Design review of the part built by this model. Coordinates are the model's own, in mm. Face numbers are marked on the shaded views. A direction names the side the tool comes from. Give positions to 0.01 mm unless a question says otherwise; leave off trailing zeros. Write each loop counter-clockwise with the first axis right and the second up, starting at its lowest first coordinate (ties: lowest second). Pieces come first, ordered by that corner, then holes. Notation, with made-up numbers: M -2.75,-17 L 27.25,-17 A23 ccw 27.25,21 Z; hole C 35,-21.5 d11. An arc over 180 degrees is marked long. Write each question's results on one line, items separated by ' | '. Start each with the question number.
from build123d import *

# Parameters (mm, degrees)
SKETCH1_W           = 20
SKETCH1_H           = 20
BOSS_EXTRUDE1_DEPTH = 6
SKETCH2_W           = 6.8
SKETCH2_H           = 20
BOSS_EXTRUDE2_DEPTH = 6
SKETCH3_W           = 7
SKETCH3_H           = 20
BOSS_EXTRUDE3_DEPTH = 15
CHAMFER1_SIZE       = 6
SKETCH4_R           = 3
CUT_EXTRUDE1_DEPTH  = 10
SKETCH5_W           = 20
SKETCH5_H           = 20
BOSS_EXTRUDE4_DEPTH = 18
CUT_EXTRUDE2_DEPTH  = 2
SKETCH9_W           = 20
SKETCH9_H           = 8.1
BOSS_EXTRUDE5_DEPTH = 23
CUT_EXTRUDE5_REACH  = 54.058
SKETCH10_R          = 3
SKETCH11_R          = 5.05
CUT_EXTRUDE6_DEPTH  = 6.1


with BuildPart() as part:
    # Sketch1 → Boss-Extrude1 (new body)
    with BuildSketch(Plane(origin=(0, 0, 0), x_dir=(1, 0, 0), z_dir=(0, 1, 0))):
        Rectangle(SKETCH1_W, SKETCH1_H)
    extrude(amount=BOSS_EXTRUDE1_DEPTH)

    # Sketch2 → Boss-Extrude2 (add)
    with BuildSketch(Plane(origin=(0, 6, 0), x_dir=(1, 0, 0), z_dir=(0, 1, 0))):
        with Locations((6.6, 0)):
            Rectangle(SKETCH2_W, SKETCH2_H)
    extrude(amount=BOSS_EXTRUDE2_DEPTH)

    # Sketch3 → Boss-Extrude3 (add)
    with BuildSketch(Plane(origin=(0, 6, 0), x_dir=(1, 0, 0), z_dir=(0, 1, 0))):
        with Locations((-6.5, 0)):
            Rectangle(SKETCH3_W, SKETCH3_H)
    extrude(amount=BOSS_EXTRUDE3_DEPTH)

    # Chamfer1
    chamfer1_edges = [part.edges().sort_by_distance(p)[0] for p in [
        (-10, 21, 0),
    ]]
    chamfer(chamfer1_edges, length=CHAMFER1_SIZE)

    # Sketch4 → Cut-Extrude1 (cut)
    with BuildSketch(Plane(origin=(-12.5, 12.5, 0), x_dir=(0, 0, 1), z_dir=(-0.7071067811865489, 0.7071067811865462, 0))):
        with Locations(Location((0, 7.432512212, 0), (0, 0, 270))):
            Circle(SKETCH4_R)
    extrude(amount=-CUT_EXTRUDE1_DEPTH, mode=Mode.SUBTRACT)

    # Sketch5 → Boss-Extrude4 (add)
    with BuildSketch(Plane.XZ):
        Rectangle(SKETCH5_W, SKETCH5_H)
    extrude(amount=BOSS_EXTRUDE4_DEPTH)

    # Sketch6 → Cut-Extrude2 (cut)
    with BuildSketch(Plane(origin=(-12.5, 12.5, 0), x_dir=(0, 0, 1), z_dir=(-0.7071067811865489, 0.7071067811865462, 0))):
        Polygon((0, 13.8411002), (-5.55, 10.636806206), (-5.55, 4.228218218), (0, 1.023924224), (5.55, 4.228218218), (5.55, 10.636806206), align=None)
    extrude(amount=-CUT_EXTRUDE2_DEPTH, mode=Mode.SUBTRACT)

    # Sketch9 → Boss-Extrude5 (add)
    with BuildSketch(Plane(origin=(10, 0, 0), x_dir=(0, 0, -1), z_dir=(1, 0, 0))):
        with Locations((0, -13.95)):
            Rectangle(SKETCH9_W, SKETCH9_H)
    boss_extrude5 = extrude(amount=BOSS_EXTRUDE5_DEPTH)

    # Sketch10 → Cut-Extrude5 (cut, up to next)
    with BuildSketch(Plane.XZ.offset(18), mode=Mode.PRIVATE) as cut_extrude5_sk1:
        with Locations(Location((25, 0, 0), (0, 0, 270))):
            Circle(SKETCH10_R)
    cut_extrude5_tool1 = extrude(cut_extrude5_sk1.sketch, amount=-CUT_EXTRUDE5_REACH, mode=Mode.PRIVATE) & part.part
    cut_extrude5 = cut_extrude5_tool1.solids().sort_by_distance((25, -18, 0))[0]
    add(cut_extrude5, mode=Mode.SUBTRACT)

    # Sketch11 → Cut-Extrude6 (cut)
    with BuildSketch(Plane(origin=(0, -9.9, 0), x_dir=(1, 0, 0), z_dir=(0, 1, 0))):
        with Locations(Location((25, 0, 0), (0, 0, 270))):
            Circle(SKETCH11_R)
    cut_extrude6 = extrude(amount=-CUT_EXTRUDE6_DEPTH, mode=Mode.SUBTRACT)

    # Mirror1: Boss-Extrude5, Cut-Extrude5, Cut-Extrude6 across plane
    add(boss_extrude5.mirror(Plane(origin=(0, 0, 0), x_dir=(0, 0, 1), z_dir=(1, 0, 0))))
    add(cut_extrude5.mirror(Plane(origin=(0, 0, 0), x_dir=(0, 0, 1), z_dir=(1, 0, 0))), mode=Mode.SUBTRACT)
    add(cut_extrude6.mirror(Plane(origin=(0, 0, 0), x_dir=(0, 0, 1), z_dir=(1, 0, 0))), mode=Mode.SUBTRACT)


solid = part.part
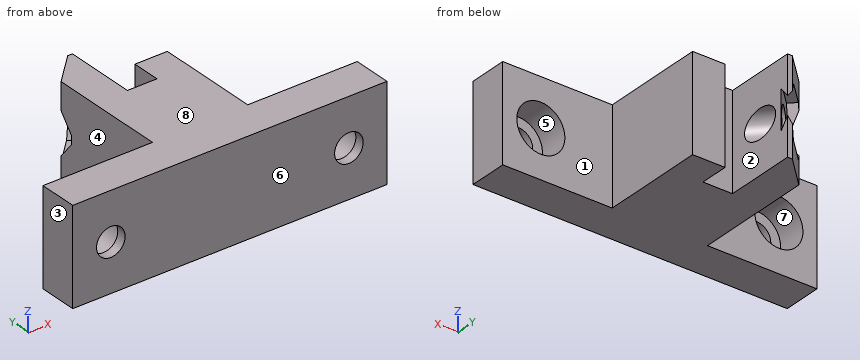
Q1. Wall thickness on line 1 along X through (y, z) = (-17.6, 0); line 2 along Z through (x, y) = (-25, -11.5); line 3 along X through (y, z) = (11, -6.25): over which ranges is each line inside the solid? List them lowest first. Write a range as from..to.
Q2. We need section B-B on x = 25. Write out the cut boundary in (y, z), and give its area (3 significant figures).
Q3. We need section C-C on z = 0. Count the separate pieces of the cut face and the enclosed holes in it, and give its area (3 significant figures).
Q4. For the marked faces 1, 2, 3 and 4, list the 3-axis set-ups (+Z, -Z, +X, -X, +Y, -Y) from which the entire face can be reached by the end or side of a thin tool; tool diameter is ignored.
Q5. We need section D-D on y = -12. Write out the cut boundary in (x, z).
Q6. The part is to be moulded in two halves that separate along Z. For the marked faces 5, 6, 7 and 8, say which applies: pulls with the +Z half, pulls with the -Z half, needs draft (parallel to the pull), parting line crosses it, or undercut.
Q7. For pin 1 Ø10 at (y, z) = (2, -4) entering from +X; pin 2 Ø10 at (y, z) = (4, -4.5) entering from -X; pin 3 Ø11.5 at (x, z) = (-25, 0) entering from +Y; pin 4 Ø7 at (x, z) = (-1.5, 2.5) entering from +Y, all flat-tipped, find the tip position at first contact; note any pin that passes through.
Q8. We need section A-A on y = 8.5. Write out the cut boundary in (x, z), and give its area (3 significant figures).
Answer sheet:
1) line 1: -33..-28, -22..22, 28..33 | line 2: -10..-5.05, 5.05..10 | line 3: -10..-3, 3.2..10
2) outline: M -18,-10 L -9.9,-10 L -9.9,-5.05 L -16,-5.05 L -16,-3 L -18,-3 Z; M -18,3 L -16,3 L -16,5.05 L -9.9,5.05 L -9.9,10 L -18,10 Z | area: 88.4 mm^2
3) separate pieces: 4 | enclosed holes: 0 | area: 790 mm^2
4) face 1: +Z, -Z, +X, +Y | face 2: +Z, -Z, +Y | face 3: +Z, -Z, -X, +Y, -Y | face 4: +Z, -Z, -X, +Y
5) outline: M -33,-10 L 33,-10 L 33,10 L -33,10 Z; hole C -25,0 d10.1; hole C 25,0 d10.1
6) face 5: undercut | face 6: needs draft | face 7: undercut | face 8: pulls with the +Z half
7) pin 1: x = 10 | pin 2: x = -10 | pin 3: y = -9.9 | pin 4: y = 21
8) outline: M -10,-10 L -3,-10 L -3,10 L -10,10 Z; M 3.2,-10 L 10,-10 L 10,10 L 3.2,10 Z | area: 276 mm^2
